Could you check a few things on this model? Use its own coordinates, in mm. Coordinates: 2 decimals unless noted, no trailing zeros. Loops run counter-clockwise (first coordinate to the right, second up) from the corner with the lowest first, then second, coordinate; pieces in that order, holes last. Notation, with made-up numbers: M -2,66 L 27,66 A19 cw 27,93 Z; hole C 49.25,-7.75 d10. An arc over 180 degrees is marked long. Return JSON: item names as keys, results as strings. Group by question number.
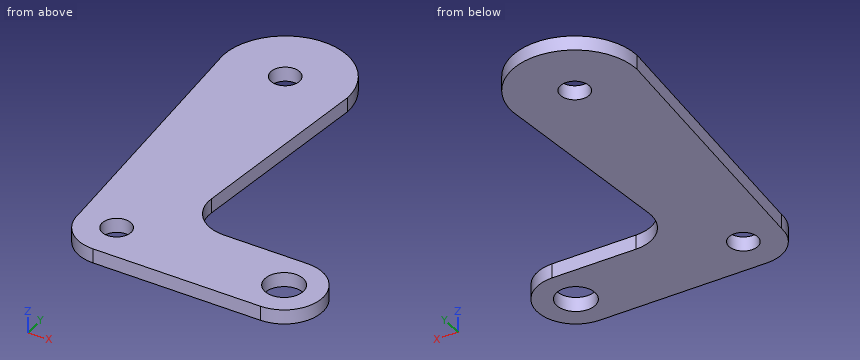
from build123d import *

# Parameters (mm, degrees)
SCHIZZO1_R          = 4
SCHIZZO1_R_2        = 3
BASE_FLANGIA3_DEPTH = 3


# Sheet-metal steps are written as plain solids
with BuildPart() as part:
    # Schizzo1 → Base-Flangia3 (new body)
    with BuildSketch(Plane.XY):
        with BuildLine():
            Line((35, -8), (0, -8))
            ThreePointArc((0, -8), (-5.656854249, -5.656854249), (-8, 0))
            Line((-8, 0), (-13, 57))
            ThreePointArc((-13, 57), (0, 70), (13, 57))
            Line((13, 57), (9.483101588, 16.695421866))
            ThreePointArc((9.483101588, 16.695421866), (11.555218404, 10.594603388), (17.452818548, 8))
            Line((17.452818548, 8), (35, 8))
            ThreePointArc((35, 8), (43, 0), (35, -8))
        make_face()
        with Locations((35, 0)):
            Circle(SCHIZZO1_R, mode=Mode.SUBTRACT)
        Circle(SCHIZZO1_R_2, mode=Mode.SUBTRACT)
        with Locations((0, 57)):
            Circle(SCHIZZO1_R_2, mode=Mode.SUBTRACT)
    extrude(amount=-BASE_FLANGIA3_DEPTH)


solid = part.part
(1) Imagine slicing it at D-D, the plane y = 21. Write out the boundary of the cut face in (x, z).
(2) Imagine slicing it at B-B, the plane x = 32. Write out the boundary of the cut face in (y, z), then the cut area to 3 significant figures.
(3) If I drill on L1, parallel to Y at x = 0, z = -2.3; L2, parallel to Y at x = 2, z = -2; L3, parallel to X at y = 2, z = -0.4, over which ranges is the centre line in solid material (lowest first)? Write a range as [from, to].
(4) Will these pins go through, and if not, where does the flat tip stop? P1, Ø1.5, axis at y = 36, z = -1.5, coming from the +X side; P2, Ø0.9, axis at x = 22.5, z = -1, coming from the +Y side.
(5) Imagine slicing it at A-A, the plane z = -2.5. Write out the boundary of the cut face in (x, y), then the cut area to 3 significant figures.
(6) Imagine slicing it at C-C, the plane x = 11. Write out the boundary of the cut face in (y, z), then the cut area to 3 significant figures.
Checks:
{
 "1": {"outline": "M -9.84,-3 L 9.86,-3 L 9.86,0 L -9.84,0 Z"},
 "2": {"outline": "M -8,-3 L -2.65,-3 L -2.65,0 L -8,0 Z; M 2.65,-3 L 8,-3 L 8,0 L 2.65,0 Z", "area": "32.1 mm²"},
 "3": {"L1": "[-8, -3], [3, 54], [60, 70]", "L2": "[-8, -2.24], [2.24, 54.76], [59.24, 69.85]", "L3": "[-8.18, -2.24], [2.24, 31.54], [38.46, 42.75]"},
 "4": {"P1": "x = 11.23", "P2": "y = 8"},
 "5": {"outline": "M -13,57 L -8,0 A8 ccw 0,-8 L 35,-8 A8 ccw 35,8 L 17.45,8 A8 cw 9.48,16.7 L 13,57 A13 ccw Z; hole C 0,0 d6; hole C 0,57 d6; hole C 35,0 d8", "area": "2,020 mm²"},
 "6": {"outline": "M -8,-3 L 11.27,-3 L 11.27,0 L -8,0 Z; M 34.08,-3 L 63.93,-3 L 63.93,0 L 34.08,0 Z", "area": "147 mm²"}
}
